Source: CAD feature listing. Evaluate the final solid. Frame: model axes, mm. Face numbers are marked on the shaded views. A direction names the side the tool comes from. Give positions to 0.01 mm unless a question says otherwise; leave off trailing zeros. Order: outer loops, then holes, each group sorted by start corner. A loop starts at its lowest first (then second) coordinate and runs counter-clockwise, first axis right, second up. Notation, with made-up numbers: (68.25, 61.5) -> (107.25, 61.5) arc R33 ccw to (107.25, 95.5) -> close; hole circle Ø10 at (-36, -13). An arc over 180 degrees is marked (long way). Use CSV: the item, a comma, the result in double quotes.
Autodesk Inventor part; units mm, degrees
ref_plane "YZ Plane" through (0, 0, 0) normal (1, 0, 0) x (0, 1, 0)
ref_plane "XZ Plane" through (0, 0, 0) normal (0, 1, 0) x (-1, 0, 0)
ref_plane "XY Plane" through (0, 0, 0) normal (0, 0, 1) x (1, 0, 0)
sketch "Sketch1" plane through (0, 0, 0) normal (0, 1, 0) x (-1, 0, 0)
  line L0 (0, 0) -> (76.2, 0)
  line L1 (76.2, 0) -> (76.2, -241.3)
  line L2 (76.2, -241.3) -> (0, -241.3)
  line L3 (0, -241.3) -> (0, 0)
  dimension "d0" = 76.2
  dimension "d1" = 241.3
extrude "Extrusion1" add sketch "Sketch1" along normal blind 19.05
sketch "Sketch3" plane through (0, 19.05, 0) normal (0, 1, 0) x (1, 0, 0)
  line L0 (-76.2, 0) -> (0, 0)
  line L1 (0, 0) -> (0, 241.3)
  line L2 (0, 241.3) -> (-76.2, 241.3)
  line L3 (-76.2, 241.3) -> (-76.2, 0)
  line L4 (-38.1, 19.05) -> (-38.1, 19.05)
  line L5 (-19.05, 38.1) -> (-19.05, 203.2)
  line L6 (-38.1, 222.25) -> (-38.1, 222.25)
  line L7 (-57.15, 203.2) -> (-57.15, 38.1)
  arc A0 (-57.15, 38.1) -> (-38.1, 19.05) centre (-38.1, 38.1) ccw
  arc A1 (-38.1, 19.05) -> (-19.05, 38.1) centre (-38.1, 38.1) ccw
  arc A2 (-19.05, 203.2) -> (-38.1, 222.25) centre (-38.1, 203.2) ccw
  arc A3 (-38.1, 222.25) -> (-57.15, 203.2) centre (-38.1, 203.2) ccw
  dimension "d11" = 19.05
  dimension "d12" = 19.05
extrude "Extrusion3" cut sketch "Sketch3" against normal blind 25.4 contours A1 A0 L7 A3 A2 L5
properties part number "Marque"
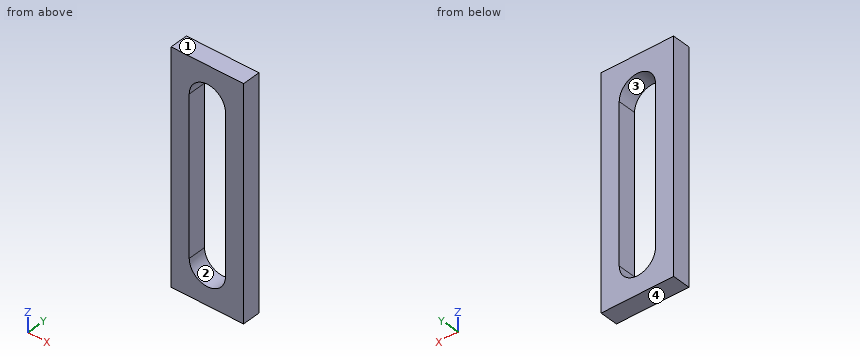
1. Pin query (flat end, axial travel): P1, Ø5.5, axis at y = 8, z = -101.5, coming from the +X side. Return the tip coordinate at first contact, or that it passes through.
Answer below:
P1,"stops at x = 0"
2. Mould query, pull axis X, two halves, no side actions, for the marked faces 1 and 2. Classes: released by +X, released by -X, zero draft, split by the parting line, or undercut.
Answer below:
face 1,"zero draft"
face 2,"undercut"
3. Access query for the marked faces 3 and 4. Directions: +Z, -Z, +X, -X, +Y, -Y. A direction counts if a zero-diameter tool reaches every point of the face in a straight line with its end or side. Return the directions, or none.
Answer below:
face 3,"+Y, -Y"
face 4,"-Z, +X, -X, +Y, -Y"
4. Section query A-A on x = -38.1. Return loops of the section in (y, z).
Answer below:
outline,"(0, -241.3) -> (19.05, -241.3) -> (19.05, -222.25) -> (0, -222.25) -> close; (0, -19.05) -> (19.05, -19.05) -> (19.05, 0) -> (0, 0) -> close"
5. Ray query, line 1 along X through (y, z) = (17.75, -97); line 2 along Z through (x, y) = (-38, 1.75); line 3 along Z through (x, y) = (-54.5, 5.5). Return the intervals inside material, ascending.
Answer below:
line 1,"x = -76.2 to -57.15, -19.05 to 0"
line 2,"z = -241.3 to -222.25, -19.05 to 0"
line 3,"z = -241.3 to -212.89, -28.41 to 0"
6. Section query B-B on z = -179. Return loops of the section in (x, y).
Answer below:
outline,"(-76.2, 0) -> (-57.15, 0) -> (-57.15, 19.05) -> (-76.2, 19.05) -> close; (-19.05, 0) -> (0, 0) -> (0, 19.05) -> (-19.05, 19.05) -> close"
7. Section query C-C on y = 13. Return loops of the section in (x, z).
Answer below:
outline,"(-76.2, -241.3) -> (0, -241.3) -> (0, 0) -> (-76.2, 0) -> close; hole (-57.15, -203.2) arc R19.05 ccw to (-19.05, -203.2) -> (-19.05, -38.1) arc R19.05 ccw to (-57.15, -38.1) -> close"
